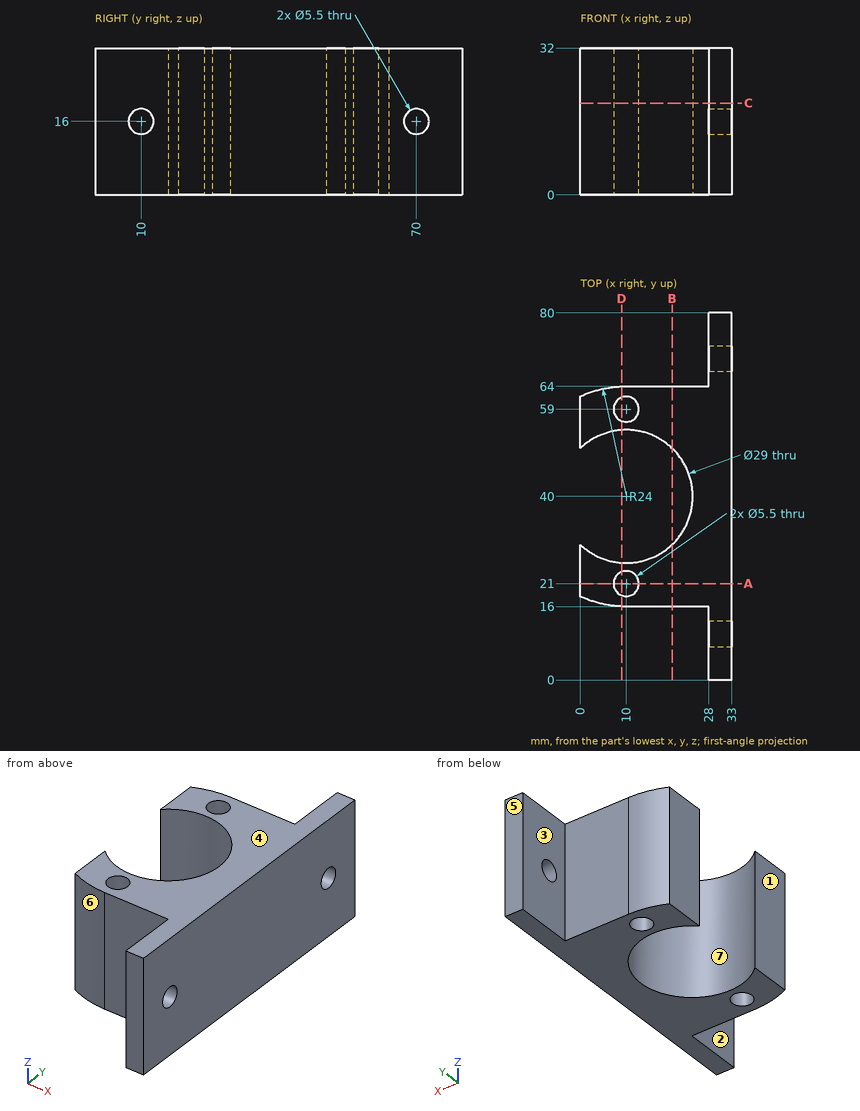
Verification items for this drawing (mm, ordinates from the low corner). A direction names the side the tool comes from. Coordinates: 2 decimals unless noted, no trailing zeros. Write each loop counter-clockwise with the first axis right and the second up, starting at its lowest first coordinate (ties: lowest second). Pieces come first, ordered by that corner, then holes. Notation, with made-up numbers: (12.25, 70.5) -> (57.25, 70.5) arc R23 cw to (57.25, 101.5) -> close; hole circle Ø1 at (47, -33.5). An arc over 180 degrees is marked (long way). One line per item, written item: value. Start each with the question number.
Q1. Cross-section at B-B on x = 20. Enter the section's corners in (y, z), and give its area (3 significant figures).
Q2. Thickness scan on L1, parallel to X at y = 59, z = 21.5; L2, parallel to Z at x = 31.8, y = 10; L3, parallel to X at y = 72, z = 19. Record the ranges inside material, lowest first. Write a range as from..to.
Q3. Go/stop test with flat-tipped pins: P1, Ø3, axis at x = 17.5, z = 16.5, coming from the -Y side; P2, Ø13, axis at y = 73, z = 17, coming from the -X side; P3, Ø4.5, axis at y = 70, z = 16, coming from the -X side; P4, Ø6, axis at x = 4.5, z = 3.5, coming from the +Y side. Record where each tip stops, or that it passes through.
Q4. Cross-section at C-C on z = 20. Enter the section's corners in (x, y).
Q5. Cross-section at A-A on y = 21. Enter the section's corners in (x, z).
Q6. Cross-section at D-D on x = 9. Enter the section's corners in (y, z).
Q7. Access from +Z, -Z, +X, -X, +Y, -Y to the whole of each face (thin tool, end or side, straight path). Record for the marked faces 1, 2 and 3.
Q8. Mould release check, pull along Y, two halves, no side actions. Record for the marked faces 4, 5, 6 and 7: pulls with the +Y half, pulls with the -Y half, needs draft (parallel to the pull), parting line crosses it, or undercut.
Checked values:
1. outline: (16, 0) -> (29.5, 0) -> (29.5, 32) -> (16, 32) -> close; (50.5, 0) -> (64, 0) -> (64, 32) -> (50.5, 32) -> close
1. area: 864 mm²
2. L1: x = 0..7.25, 12.75..33
2. L2: z = 0..13.25, 18.75..32
2. L3: x = 28..33
3. P1: stops at y = 16
3. P2: stops at x = 28
3. P3: passes through
3. P4: stops at y = 63.87
4. outline: (0, 18.18) arc R24 ccw to (10, 16) -> (28, 16) -> (28, 0) -> (33, 0) -> (33, 80) -> (28, 80) -> (28, 64) -> (10, 64) arc R24 ccw to (0, 61.82) -> (0, 50.5) arc R14.5 cw (long way) to (0, 29.5) -> close; hole circle Ø5.5 at (10, 21); hole circle Ø5.5 at (10, 59)
5. outline: (0, 0) -> (7.25, 0) -> (7.25, 32) -> (0, 32) -> close; (12.75, 0) -> (33, 0) -> (33, 32) -> (12.75, 32) -> close
6. outline: (16.02, 0) -> (18.44, 0) -> (18.44, 32) -> (16.02, 32) -> close; (23.56, 0) -> (25.53, 0) -> (25.53, 32) -> (23.56, 32) -> close; (54.47, 0) -> (56.44, 0) -> (56.44, 32) -> (54.47, 32) -> close; (61.56, 0) -> (63.98, 0) -> (63.98, 32) -> (61.56, 32) -> close
7. face 1: +Z, -Z, -X, +Y, -Y
7. face 2: +Z, -Z, -X, -Y
7. face 3: +Z, -Z, -X, +Y
8. face 4: needs draft
8. face 5: pulls with the +Y half
8. face 6: pulls with the -Y half
8. face 7: undercut
